```python
from build123d import *

# Parameters (mm, degrees)
BOSS_EXTRUDE1_DEPTH = 25
SKETCH4_R           = 7.25
CUT_EXTRUDE1_DEPTH  = 25


with BuildPart() as part:
    # Sketch1 → Boss-Extrude1 (new body)
    with BuildSketch(Plane.XY):
        with BuildLine():
            Line((150, 0), (150, 6.5))
            Line((150, 6.5), (40, 6.5))
            Line((40, 6.5), (40, 26.5))
            ThreePointArc((40, 26.5), (0, 66.5), (-40, 26.5))
            Line((-40, 26.5), (-40, 6.5))
            Line((-40, 6.5), (-150, 6.5))
            Line((-150, 6.5), (-150, 0))
            Line((-150, 0), (-33.5, 0))
            Line((-33.5, 0), (-33.5, 26.5))
            ThreePointArc((-33.5, 26.5), (0, 60), (33.5, 26.5))
            Line((33.5, 26.5), (33.5, 0))
            Line((33.5, 0), (150, 0))
        make_face()
    extrude(amount=BOSS_EXTRUDE1_DEPTH)

    # Sketch4 → Cut-Extrude1 (cut)
    with BuildSketch(Plane(origin=(0, 0, 0), x_dir=(1, 0, 0), z_dir=(0, 1, 0))):
        with Locations((-60, -12.5)):
            Circle(SKETCH4_R)
        with Locations((-100, -12.5)):
            Circle(SKETCH4_R)
        with Locations(Location((60, -12.5, 0), (0, 0, 90))):
            Circle(SKETCH4_R)
        with Locations(Location((100, -12.5, 0), (0, 0, 90))):
            Circle(SKETCH4_R)
    extrude(amount=CUT_EXTRUDE1_DEPTH, mode=Mode.SUBTRACT)


solid = part.part
```
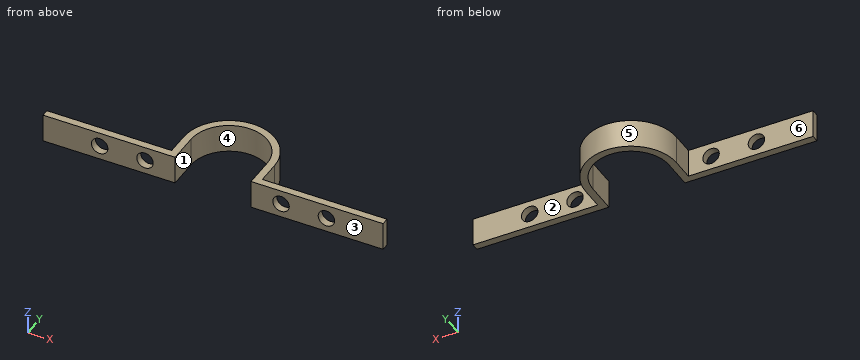
Geometry check sheet. Reference: the model listing, model coordinates, mm. Face numbers are marked on the shaded views. A direction names the side the tool comes from. Round coordinates to 2 decimals unless told otherwise and drop trailing zeros. Loops run counter-clockwise (first coordinate to the right, second up) from the corner with the lowest first, then second, coordinate; pieces in that order, holes last. Notation, with made-up numbers: (54, -31) - (72, -31) arc R15 ccw to (72, -23) - close; hole circle Ø7 at (42.5, 39). An arc over 180 degrees is marked (long way). Write item = value, one per line. Start each with the question number.
1. Section check A-A on y = 13.5. Enter the section's corners in (x, z).
2. Section check D-D on x = -124. Enter the section's corners in (y, z), then the cut area to 4 significant figures.
3. Section check B-B on x = -60. Enter the section's corners in (y, z), then the cut area to 4 significant figures.
4. Mould release check, pull along X, two halves, no side actions. Record for the marked faces 4, 5 and 6: released by +X, released by -X, zero draft, split by the parting line, or undercut.
5. Set-up check for the marked faces 1, 2 and 3: record each of +Z, -Z, +X, -X, +Y, -Y from which the full face is reachable in a straight line by a thin tool's end or side.
6. Depth check by flat-ended pin: pin 1 (3 mm diameter, centred on x = -1.5, z = 6.5, fed in from +Y); pin 2 (5 mm diameter, centred on x = 73.5, z = 3.5, fed in from -Y); pin 3 (5 mm diameter, centred on x = -76, z = 6, fed in from +Y); pin 4 (8 mm diameter, centred on y = 48.5, z = 20.5, fed in from +X). Enter the tip coordinate at first touch or a pass-through.
7. Section check C-C on z = 12.5. Enter the section's corners in (x, y).
8. Thickness scan on line 1 (X direction, y = 3.5, z = 12.5); line 2 (Z direction, x = -60, y = 2.75); line 3 (X direction, y = 12, z = 12.5). Record the ranges inside material, lowest first.
Working result:
q1.outline = (-40, 0) - (-33.5, 0) - (-33.5, 25) - (-40, 25) - close; (33.5, 0) - (40, 0) - (40, 25) - (33.5, 25) - close
q2.outline = (0, 0) - (6.5, 0) - (6.5, 25) - (0, 25) - close
q2.area = 162.5 mm^2
q3.outline = (0, 0) - (6.5, 0) - (6.5, 5.25) - (0, 5.25) - close; (0, 19.75) - (6.5, 19.75) - (6.5, 25) - (0, 25) - close
q3.area = 68.25 mm^2
q4.face_4 = undercut
q4.face_5 = split by the parting line
q4.face_6 = zero draft
q5.face_1 = +Z, -Z, -Y
q5.face_2 = +Z, -Z, +X, +Y
q5.face_3 = +Z, -Z, +X, -X, -Y
q6.pin_1 = 66.5
q6.pin_2 = 0
q6.pin_3 = 6.5
q6.pin_4 = 35.72
q7.outline = (-150, 0) - (-107.25, 0) - (-107.25, 6.5) - (-150, 6.5) - close; (-92.75, 0) - (-67.25, 0) - (-67.25, 6.5) - (-92.75, 6.5) - close; (-52.75, 0) - (-33.5, 0) - (-33.5, 26.5) arc R33.5 cw to (33.5, 26.5) - (33.5, 0) - (52.75, 0) - (52.75, 6.5) - (40, 6.5) - (40, 26.5) arc R40 ccw to (-40, 26.5) - (-40, 6.5) - (-52.75, 6.5) - close; (67.25, 0) - (92.75, 0) - (92.75, 6.5) - (67.25, 6.5) - close; (107.25, 0) - (150, 0) - (150, 6.5) - (107.25, 6.5) - close
q8.line_1 = -150 to -107.25, -92.75 to -67.25, -52.75 to -33.5, 33.5 to 52.75, 67.25 to 92.75, 107.25 to 150
q8.line_2 = 0 to 5.25, 19.75 to 25
q8.line_3 = -40 to -33.5, 33.5 to 40
